```python
from build123d import *

# Parameters (mm, degrees)
F1_DEPTH = 103.759
F2_W     = 5.207
F2_H     = 2.8575
F2_H_2   = 16.2052
F2_H_3   = 2.9408035447
F3_DEPTH = 2.9972
F4_R     = 2.54
F5_DEPTH = 7.239
F6_R     = 3.175
F7_DEPTH = 5.08


with BuildPart() as f1:
    # F0 (on Right) → F1 (new body)
    with BuildSketch(Plane.YZ):
        Polygon((0, 1.524), (0, 0), (16.2052, 0), (16.2052, 1.524), (19.0627, 4.3815), (16.2052, 7.239), (0, 7.239), (-2.8575, 4.3815), align=None)
    extrude(amount=F1_DEPTH)

    # F2 (on face) → F3 (cut)
    with BuildSketch(Plane.XY.offset(7.239)):
        with Locations((7.3025, -1.42875)):
            Rectangle(F2_W, F2_H)
        Polygon((4.699, 16.2052), (4.699, 8.1026), (4.699, 0), (9.906, 0), (9.906, 16.2052), align=None)
        with Locations((7.3025, 17.63395)):
            Rectangle(F2_W, F2_H)
        with Locations((17.2085, 17.63395)):
            Rectangle(F2_W, F2_H)
        with Locations((17.2085, 8.1026)):
            Rectangle(F2_W, F2_H_2)
        with Locations((17.2085, -1.42875)):
            Rectangle(F2_W, F2_H)
        with Locations((27.1145, 17.63395)):
            Rectangle(F2_W, F2_H)
        with Locations((27.1145, 8.1026)):
            Rectangle(F2_W, F2_H_2)
        with Locations((27.1145, -1.42875)):
            Rectangle(F2_W, F2_H)
        with Locations((37.0205, 17.63395)):
            Rectangle(F2_W, F2_H)
        with Locations((37.0205, 8.1026)):
            Rectangle(F2_W, F2_H_2)
        with Locations((37.0205, -1.42875)):
            Rectangle(F2_W, F2_H)
        with Locations((46.9265, 17.63395)):
            Rectangle(F2_W, F2_H)
        with Locations((46.9265, 8.1026)):
            Rectangle(F2_W, F2_H_2)
        with Locations((46.9265, -1.42875)):
            Rectangle(F2_W, F2_H)
        with Locations((56.8325, 17.63395)):
            Rectangle(F2_W, F2_H)
        with Locations((56.8325, 8.1026)):
            Rectangle(F2_W, F2_H_2)
        with Locations((56.8325, -1.42875)):
            Rectangle(F2_W, F2_H)
        with Locations((66.7385, 17.63395)):
            Rectangle(F2_W, F2_H)
        with Locations((66.7385, 8.1026)):
            Rectangle(F2_W, F2_H_2)
        with Locations((66.7385, -1.42875)):
            Rectangle(F2_W, F2_H)
        with Locations((76.6445, 17.63395)):
            Rectangle(F2_W, F2_H)
        with Locations((76.6445, 8.1026)):
            Rectangle(F2_W, F2_H_2)
        with Locations((76.6445, -1.42875)):
            Rectangle(F2_W, F2_H)
        with Locations((86.5505, -1.42875)):
            Rectangle(F2_W, F2_H)
        with Locations((86.5505, 8.1026)):
            Rectangle(F2_W, F2_H_2)
        with Locations((86.5505, 17.63395)):
            Rectangle(F2_W, F2_H)
        with Locations((96.4565, 17.6756017723)):
            Rectangle(F2_W, F2_H_3)
        with Locations((96.4565, 8.1026)):
            Rectangle(F2_W, F2_H_2)
        with Locations((96.4565, -1.4704017723)):
            Rectangle(F2_W, F2_H_3)
    extrude(amount=-F3_DEPTH, mode=Mode.SUBTRACT)

    # F4 (on face) → F5 (cut)
    with BuildSketch(Plane(origin=(0, 0, 0), x_dir=(1, 0, 0), z_dir=(0, 0, -1))):
        with Locations((93.4012121817, -8.3558605984)):
            Circle(F4_R)
        with Locations((10.16, -8.1026)):
            Circle(F4_R)
    extrude(amount=-F5_DEPTH, mode=Mode.SUBTRACT)

    # F6 (on face) → F7 (cut)
    with BuildSketch(Plane.XY.offset(7.239)):
        with Locations((93.4012121817, 8.3558605984)):
            Circle(F6_R)
        with Locations((10.16, 8.1026)):
            Circle(F6_R)
    extrude(amount=-F7_DEPTH, mode=Mode.SUBTRACT)


solid = f1.part
```
Input: part model. Units: mm. Frame: model coordinates. A direction names the side the tool comes from. Coordinates: 2 decimals unless noted, no trailing zeros. Answer in a Markdown table with one row per item.
(1) Material intervals for L1, parallel to X at y = 8, z = 3; L2, parallel to X at y = 8.5, z = 1.75; L3, parallel to Y at x = 10.16, z = 1.65, sorted ascending. Write a range as from..to.
Model answer:
| item | result |
|---|---|
| L1 | x = 0..6.99, 13.33..90.25, 96.56..103.76 |
| L2 | x = 0..7.65, 12.67..90.87, 95.94..103.76 |
| L3 | y = -0.13..5.56, 10.64..16.33 |
(2) Set-up query: faces 1 (the face through (19.812, 8, 6)), 2 (the face through (12.223, 17.654, 5.79)). Return all of +Z, -Z, +X, -X, +Y, -Y with unobstructed straight access to the full face (end or side cutting, diameter ignored); none if empty.
Model answer:
| item | result |
|---|---|
| face 1 | +Z, +Y, -Y |
| face 2 | +Z, +X, -X, +Y |
(3) Cut plane A-A on z = 5.5. Count the separate pieces of the cut face and the enclosed holes in it, plus the area to 3 significant figures.
Model answer:
| item | result |
|---|---|
| separate pieces | 11 |
| enclosed holes | 0 |
| area | 981 mm² |
(4) Mould query, pull axis X, two halves, no side actions, for faces 3 (the face through (101.377, 17.654, 5.79)), 4 (the face through (9.906, 2, 6)). Classes: pulls with the +X half, pulls with the -X half, needs draft (parallel to the pull), parting line crosses it, or undercut.
Model answer:
| item | result |
|---|---|
| face 3 | needs draft |
| face 4 | undercut |
(5) Pin query (flat end, axial travel): P1, Ø1.6, axis at x = 36, y = 5.5, coming from the +Z side; P2, Ø1.7, axis at x = 49.5, z = 0.5, coming from the -Y side; P3, Ø1.7, axis at x = 66, z = 0.5, coming from the +Y side. Return the tip coordinate at first contact, or that it passes through.
Model answer:
| item | result |
|---|---|
| P1 | stops at z = 4.24 |
| P2 | stops at y = 0 |
| P3 | stops at y = 16.21 |
